For this review, take the finished solid that the model builds, in its own axes (mm). Face numbers are marked on the shaded views. A direction names the side the tool comes from. Coordinates: 2 decimals unless noted, no trailing zeros.
```python
from build123d import *

# Parameters (mm, degrees)
SKETCH1_R                       = 1.225
BOSS_EXTRUDE1_DEPTH             = 7.5
CUT_EXTRUDE2_DEPTH              = 1.725
BOSS_EXTRUDE3_REACH             = 43.137
BOSS_EXTRUDE3_DIRECTION_2_REACH = 43.137
FILLET5_R                       = 5
FILLET6_R                       = 4
FILLET7_R                       = 2
FILLET8_R                       = 0.4


with BuildPart() as part:
    # Sketch1 → Boss-Extrude1 (new, symmetric)
    with BuildSketch(Plane.XY):
        Polygon((-6, -4), (6, -4), (6, 4), (-2, 40), (-6, 40), align=None)
        with Locations((-2.5, 0)):
            Circle(SKETCH1_R, mode=Mode.SUBTRACT)
        with Locations((2.5, 0)):
            Circle(SKETCH1_R, mode=Mode.SUBTRACT)
    extrude(amount=BOSS_EXTRUDE1_DEPTH, both=True)

    # Sketch4 → Cut-Extrude2 (cut, symmetric)
    with BuildSketch(Plane.XY):
        with BuildLine():
            Line((-3.05, 3), (3.05, 3))
            ThreePointArc((3.05, 3), (5.489518395, 1.989518395), (6.5, -0.45))
            Line((6.5, -0.45), (6.5, -4))
            Line((6.5, -4), (-6.5, -4))
            Line((-6.5, -4), (-6.5, -0.45))
            ThreePointArc((-6.5, -0.45), (-5.489518395, 1.989518395), (-3.05, 3))
        make_face()
    extrude(amount=CUT_EXTRUDE2_DEPTH, both=True, mode=Mode.SUBTRACT)

    # Boss-Extrude3: up to this face of the body (flat: up to its plane)
    boss_extrude3_end = Plane(part.part.faces().sort_by_distance((-1.281464988, 14.60870086, 7.5))[0])
    # Sketch6 → Boss-Extrude3 (add, up to the picked face)
    with BuildSketch(Plane.XY, mode=Mode.PRIVATE) as boss_extrude3_sk1:
        Polygon((-6, 40), (-6, 3), (-8, 5), (-8, 7), (-7, 8), (-7, 10), (-8, 11), (-8, 13), (-7, 14), (-7, 16), (-8, 17), (-8, 19), (-7, 20), (-7, 22), (-8, 23), (-8, 25), (-7, 26), (-7, 28), (-8, 29), (-8, 31), (-7, 32), (-7, 34), (-8, 35), (-8, 40), align=None)
    boss_extrude3_tool1 = split(extrude(boss_extrude3_sk1.sketch, amount=BOSS_EXTRUDE3_REACH, mode=Mode.PRIVATE), bisect_by=boss_extrude3_end, keep=Keep.BOTH, mode=Mode.PRIVATE)
    add(boss_extrude3_tool1.solids().sort_by(Axis((-6.842105, 22.25731, 0), (0, 0, 1)))[0])

    # Boss-Extrude3 direction 2: up to this face of the body (flat: up to its plane)
    boss_extrude3_direction_2_end = Plane(part.part.faces().sort_by_distance((-1.281464988, 14.60870086, -7.5))[0])
    # Sketch6 → Boss-Extrude3 direction 2 (add, up to the picked face)
    with BuildSketch(Plane.XY, mode=Mode.PRIVATE) as boss_extrude3_direction_2_sk1:
        Polygon((-6, 40), (-6, 3), (-8, 5), (-8, 7), (-7, 8), (-7, 10), (-8, 11), (-8, 13), (-7, 14), (-7, 16), (-8, 17), (-8, 19), (-7, 20), (-7, 22), (-8, 23), (-8, 25), (-7, 26), (-7, 28), (-8, 29), (-8, 31), (-7, 32), (-7, 34), (-8, 35), (-8, 40), align=None)
    boss_extrude3_direction_2_tool1 = split(extrude(boss_extrude3_direction_2_sk1.sketch, amount=-BOSS_EXTRUDE3_DIRECTION_2_REACH, mode=Mode.PRIVATE), bisect_by=boss_extrude3_direction_2_end, keep=Keep.BOTH, mode=Mode.PRIVATE)
    add(boss_extrude3_direction_2_tool1.solids().sort_by(Axis((-6.842105, 22.25731, 0), (0, 0, -1)))[0])

    # Fillet5
    fillet5_edges = [part.edges().sort_by_distance(p)[0] for p in [
        (-2, 40, 0),
    ]]
    fillet(fillet5_edges, radius=FILLET5_R)

    # Fillet6
    fillet6_edges = [part.edges().sort_by_distance(p)[0] for p in [
        (6, -4, -4.6125),
        (-6, -4, -4.6125),
        (6, -4, 4.6125),
        (-6, -4, 4.6125),
    ]]
    fillet(fillet6_edges, radius=FILLET6_R)

    # Fillet7
    fillet7_edges = [part.edges().sort_by_distance(p)[0] for p in [
        (-2.882221064, 38.900209061, -7.5),
        (-2.882221064, 38.900209061, 7.5),
        (2.435038635, 20.042326145, -7.5),
        (2.435038635, 20.042326145, 7.5),
        (-7.005429016, 40, -7.5),
        (-7.005429016, 40, 7.5),
    ]]
    fillet(fillet7_edges, radius=FILLET7_R)

    # Fillet8
    fillet8_edges = [part.edges().sort_by_distance(p)[0] for p in [
        (6, 1.338854382, 0),
        (-6, 1.338854382, 0),
    ]]
    fillet(fillet8_edges, radius=FILLET8_R)


solid = part.part
```
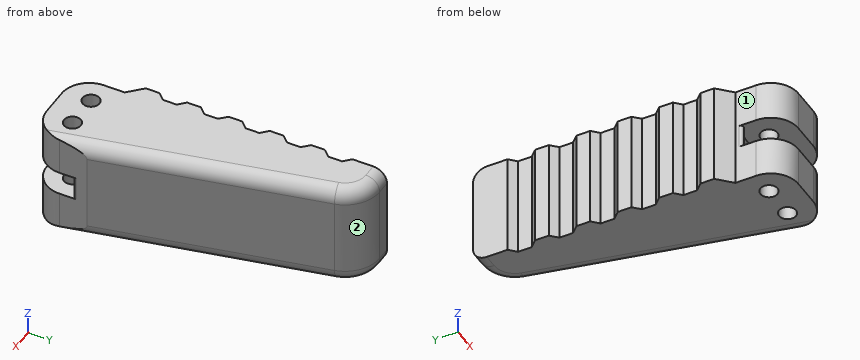
Q1. Clearance check with flat-ended pins moving along their axes: pin 1 Ø8 at (y, z) = (25.5, -5) entering from +X; pin 2 Ø3.5 at (y, z) = (1, -3) entering from -X; pin 3 Ø1.5 at (x, z) = (-4, 5) entering from +Y. State where each tip first meets the part, or that it passes through.
Ans:
pin 1: stops at x = 2.11
pin 2: stops at x = -6
pin 3: stops at y = 39.84
Q2. Add section A-A (z = 2.75). Give the number of separate pieces and of enclosed holes in the cut face, then the cut area to 3 significant figures.
Ans:
separate pieces: 1
enclosed holes: 2
area: 422 mm2
Q3. For probe 1 along X at (y, z) = (0, -4.9) (3 decimals); probe 2 along Z at (x, y) = (3.5, -1) (3 decimals); probe 3 along Y at (x, z) = (-2.75, -4.25), list the stretches that pass through material, from the lowest coordinate up.
Ans:
probe 1: x = -6 to -3.725, -1.275 to 1.275, 3.725 to 6
probe 2: z = -7.5 to -1.725, 1.725 to 7.5
probe 3: y = -3.93 to -1.2, 1.2 to 38.79
Q4. Tool access review of the marked faces 1 and 2: name each direction out of +Z, -Z, +X, -X, +Y, -Y from which nothing blocks a thin tool from reaching the whole face with its end or side.
Ans:
face 1: +Z, -Z, -X, -Y
face 2: +Z, -Z, +X, +Y
